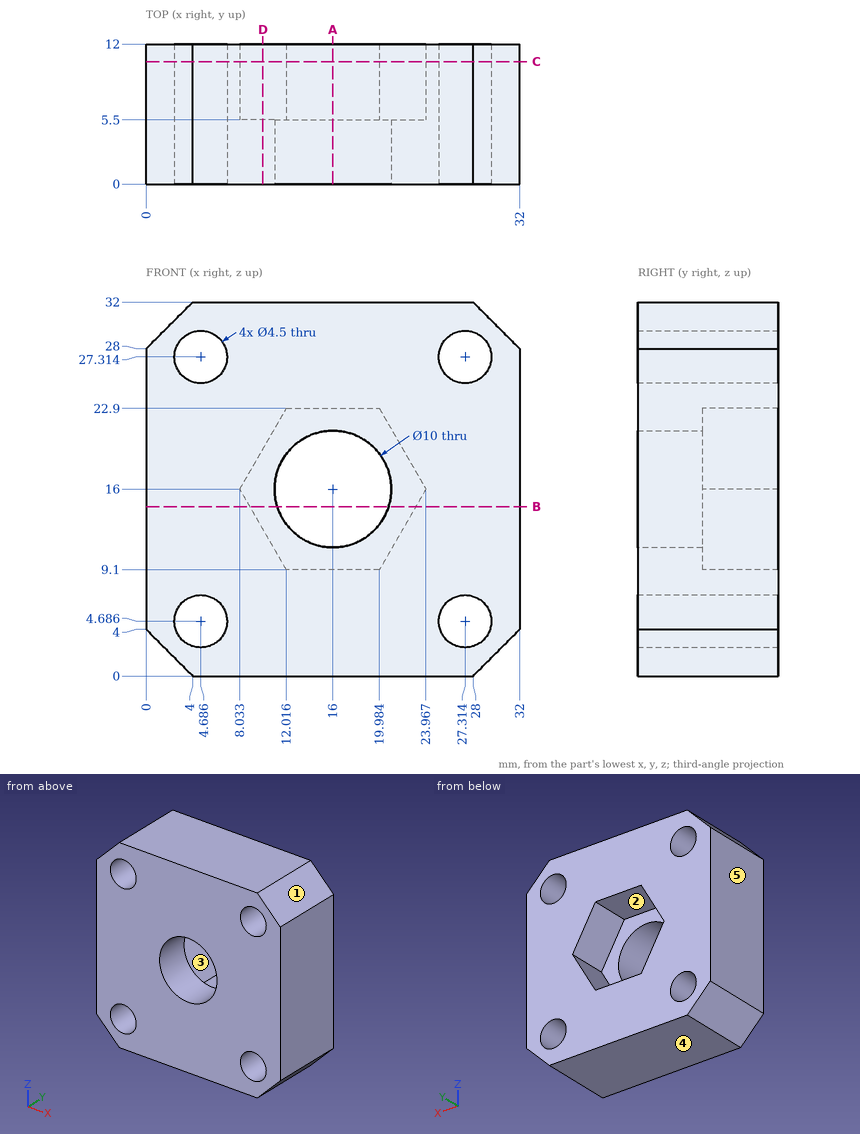
Study the drawing (mm; zero at the part's minimum x, y, z) and answer. A direction names the side the tool comes from. Round coordinates to 2 decimals unless told otherwise and drop trailing zeros. Write each loop counter-clockwise with the first axis right and the second up, starting at its lowest first coordinate (ties: lowest second). Pieces come first, ordered by that corner, then holes. Notation, with made-up numbers: (-10.5, -38.75) - (33.5, -38.75) arc R25 ccw to (33.5, -22.75) - close; hole circle Ø7 at (27.25, -4). An arc over 180 degrees is marked (long way). Use a Markdown table: item, result. Add a question column.
1. The part is cut by section C-C (y = 10.5). Write down the section's boundary in (x, z).
2. Consider line 1 (Z direction, x = 6.5, y = 5.5) (1 decimal); line 2 (Z direction, x = 27, y = 2.75) (1 decimal); line 3 (Z direction, x = 16, y = 2.5). Determine where each line is inside the solid, lowest interval first.
3. The part is cut by section A-A (x = 16). Write down the section's boundary in (y, z), and give its area (3 significant figures).
4. The part is cut by section D-D (x = 10). Write down the section's boundary in (y, z).
5. Flat-ended cylindrical pins translate along their axes: P1, Ø12, axis at x = 16.5, z = 25.5, coming from the -Y side; P2, Ø13, axis at x = 16, z = 16, coming from the +Y side. Find the tip coordinate at first contact, or state that the pin passes through.
6. A tool of negligible diameter and unlimited length cuts with its end or side. For the marked faces 1 and 2, from which of +Z, -Z, +X, -X, +Y, -Y can it reach the whole face along a straight path? Write none if from no direction.
7. For a pull along X with two mould halves and no side action, classify the marked faces 3, 4 and 5 as +X half, -X half, draft (parallel to the pull), parting line (faces both ways), or undercut.
8. The part is cut by section B-B (z = 14.5). Write down the section's boundary in (x, y).
Reported:
| question | item | result |
|---|---|---|
| 1 | outline | (0, 4) - (4, 0) - (28, 0) - (32, 4) - (32, 28) - (28, 32) - (4, 32) - (0, 28) - close; hole circle Ø4.5 at (4.69, 4.69); hole circle Ø4.5 at (4.69, 27.31); hole (8.03, 16) - (12.02, 9.1) - (19.98, 9.1) - (23.97, 16) - (19.98, 22.9) - (12.02, 22.9) - close; hole circle Ø4.5 at (27.31, 4.69); hole circle Ø4.5 at (27.31, 27.31) |
| 2 | line 1 | 0 to 3.4, 6 to 26, 28.6 to 32 |
| 2 | line 2 | 0 to 2.5, 6.9 to 25.1, 29.5 to 32 |
| 2 | line 3 | 0 to 11, 21 to 32 |
| 3 | outline | (0, 0) - (12, 0) - (12, 9.1) - (5.5, 9.1) - (5.5, 11) - (0, 11) - close; (0, 21) - (5.5, 21) - (5.5, 22.9) - (12, 22.9) - (12, 32) - (0, 32) - close |
| 3 | area | 239 mm^2 |
| 4 | outline | (0, 0) - (12, 0) - (12, 12.59) - (5.5, 12.59) - (5.5, 19.41) - (12, 19.41) - (12, 32) - (0, 32) - close |
| 5 | P1 | y = 0 |
| 5 | P2 | y = 5.5 |
| 6 | face 1 | +Z, +X, +Y, -Y |
| 6 | face 2 | +Y |
| 7 | face 3 | undercut |
| 7 | face 4 | draft |
| 7 | face 5 | -X half |
| 8 | outline | (0, 0) - (11.23, 0) - (11.23, 5.5) - (8.9, 5.5) - (8.9, 12) - (0, 12) - close; (20.77, 0) - (32, 0) - (32, 12) - (23.1, 12) - (23.1, 5.5) - (20.77, 5.5) - close |
